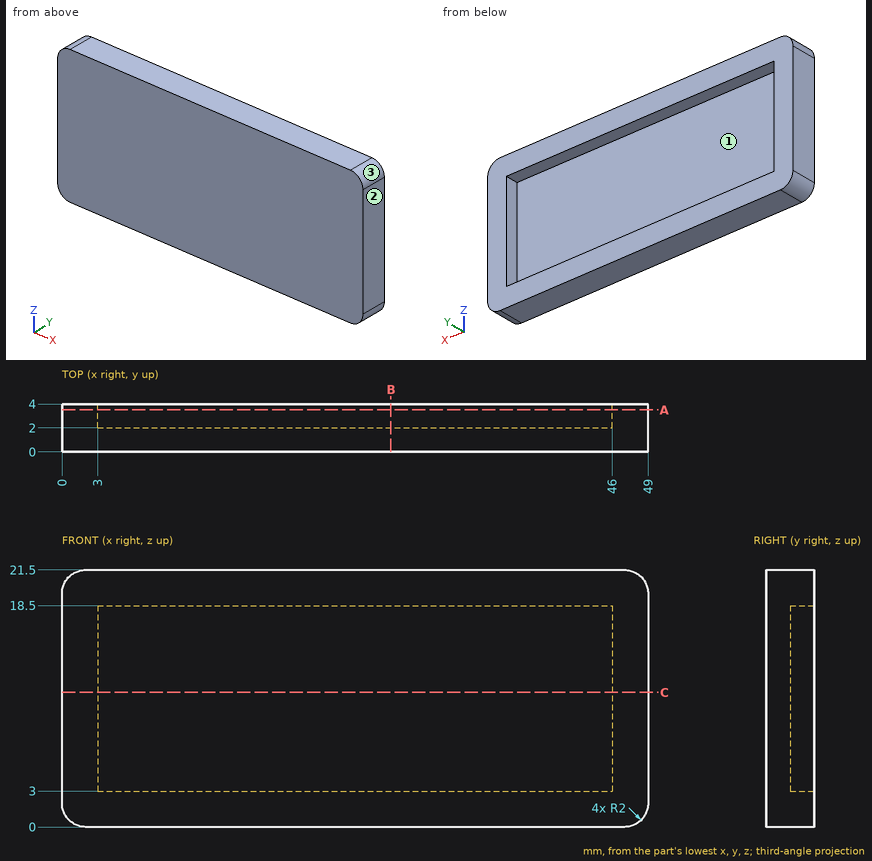
Job drawing, mm, ordinate dimensions from the low corner. One solid piece. Round coordinates to 2 decimals unless told otherwise and drop trailing zeros. Write each loop counter-clockwise with the first axis right and the second up, starting at its lowest first coordinate (ties: lowest second). Pieces come first, ordered by that corner, then holes.
1) Band-saw the part on B-B, the plane x = 27.5. List the corners of the cut face in (y, z), and give its area (3 significant figures).
2) Band-saw the part on C-C, the plane z = 11.25. List the corners of the cut face in (x, y), and give its area (3 significant figures).
3) Pin check, flat tip, straight feed: pin 1 (3 mm diameter, centred on x = 36, z = 16.5, fed in from +Y). Stop position of the tip, or through.
4) Drill centre lines: probe 1 along X at (y, z) = (2.9, 4); probe 2 along Z at (x, y) = (20, 3.2); probe 3 along Y at (x, z) = (7, 7.5). Where is each one in solid material? Low to high.
5) Mould opens along Z. For the marked faces 1, 2 and 3 say: +Z half, -Z half, draft (parallel to the pull), parting line (faces both ways), or undercut.
6) Band-saw the part on A-A, the plane y = 3.5. List the corners of the cut face in (x, z).
Ans:
1. outline: (0, 0) - (4, 0) - (4, 3) - (2, 3) - (2, 18.5) - (4, 18.5) - (4, 21.5) - (0, 21.5) - close
1. area: 55.0 mm2
2. outline: (0, 0) - (49, 0) - (49, 4) - (46, 4) - (46, 2) - (3, 2) - (3, 4) - (0, 4) - close
2. area: 110 mm2
3. pin 1: stops at y = 2
4. probe 1: x = 0 to 3, 46 to 49
4. probe 2: z = 0 to 3, 18.5 to 21.5
4. probe 3: y = 0 to 2
5. face 1: undercut
5. face 2: draft
5. face 3: +Z half
6. outline: (0, 2) arc R2 ccw to (2, 0) - (47, 0) arc R2 ccw to (49, 2) - (49, 19.5) arc R2 ccw to (47, 21.5) - (2, 21.5) arc R2 ccw to (0, 19.5) - close; hole (3, 3) - (46, 3) - (46, 18.5) - (3, 18.5) - close
